Input: part model. Units: mm. Frame: model coordinates. Face numbers are marked on the shaded views. Give positions to 0.01 mm unless a question says otherwise; leave off trailing zeros. Write each loop counter-clockwise with the first axis right and the second up, starting at its lowest first coordinate (ties: lowest second). Pieces come first, ordered by that corner, then holes. Notation, with made-up numbers: (56, -8) -> (96, -8) arc R18 ccw to (96, 0) -> close; hole circle Ø8 at (-40, -22.5). An arc over 180 degrees is marked (long way). Answer as a JSON object with one key per item and string values. Group by question number.
from build123d import *

# Parameters (mm, degrees)
SKETCH1_R               = 26
SKETCH1_R_2             = 23.9
BOSS_EXTRUDE1_DEPTH     = 300
SKETCH3_R               = 2.75
CUT_EXTRUDE2_DEPTH      = 27
CIRPATTERN1_COUNT       = 3
SKETCH5_R               = 2.75
CUT_EXTRUDE3_DEPTH      = 27.0000001
CUT_EXTRUDE3_DEPTH_BACK = 27.0000001


with BuildPart() as part:
    # Sketch1 → Boss-Extrude1 (new body)
    with BuildSketch(Plane(origin=(0, 0, 0), x_dir=(1, 0, 0), z_dir=(0, 1, 0))):
        Circle(SKETCH1_R)
        Circle(SKETCH1_R_2, mode=Mode.SUBTRACT)
    extrude(amount=BOSS_EXTRUDE1_DEPTH)

    # Sketch3 → Cut-Extrude2 (cut, through all)
    with BuildSketch(Plane.XY):
        with Locations((0, 6)):
            Circle(SKETCH3_R)
        with Locations((0, 187)):
            Circle(SKETCH3_R)
    cut_extrude2 = extrude(amount=-CUT_EXTRUDE2_DEPTH, mode=Mode.SUBTRACT)

    # CirPattern1: Cut-Extrude2 ×3 about axis
    cirpattern1_axis = Axis((0, 300, 0), (0, -1, 0))
    for i in range(1, CIRPATTERN1_COUNT):
        add(cut_extrude2.rotate(cirpattern1_axis, i * 360 / CIRPATTERN1_COUNT), mode=Mode.SUBTRACT)

    # Sketch5 → Cut-Extrude3 (cut, two sides)
    with BuildSketch(Plane(origin=(0, 0, 0), x_dir=(0, 0, -1), z_dir=(1, 0, 0))) as cut_extrude3_sk:
        with Locations((0, 187)):
            Circle(SKETCH5_R)
        with Locations((0, 6)):
            Circle(SKETCH5_R)
    extrude(amount=CUT_EXTRUDE3_DEPTH, mode=Mode.SUBTRACT)
    extrude(cut_extrude3_sk.sketch, amount=-CUT_EXTRUDE3_DEPTH_BACK, mode=Mode.SUBTRACT)


solid = part.part
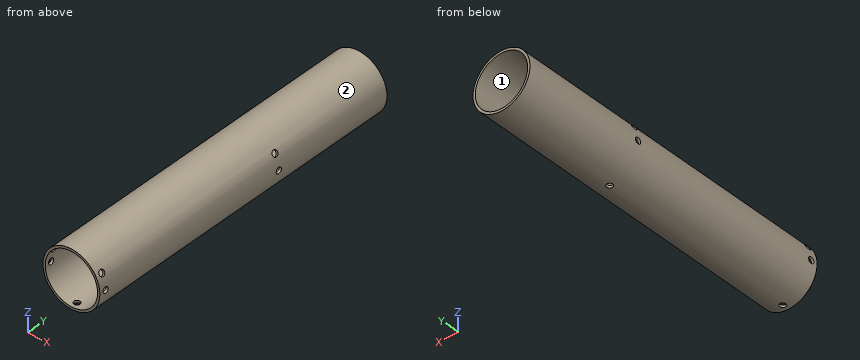
1. Line query: line 1 (Y direction, x = 0, z = -25.4); line 2 (X direction, y = 164, z = 0). Output: solid intervals per line, ascending.
2. Section D-D (z = -11). Return the cut outline in (x, y), plus the area to 3 significant figures.
3. Section C-C (y = 187). Return the cut outline in (x, z), plus the area to 3 significant figures.
4. Mould query, pull axis X, two halves, no side actions, for the marked faces 1 and 2. Classes: pulls with the +X half, pulls with the -X half, needs draft (parallel to the pull), parting line crosses it, or undercut.
5. Contact query for flat-ended pins moving along their axis: pin 1 Ø9 at (x, y) = (0, 187) entering from +Z; pin 2 Ø6.5 at (y, z) = (187, 0) entering from -X; pin 3 Ø6 at (y, z) = (127, 5) entering from +X; pin 4 Ø1 at (x, y) = (18.5, 215.5) entering from -Z. Output: stop coordinate, or through.
6. Section A-A (x = 0). Return the cut outline in (y, z).
7. Section B-B (z = 0). Return the cut outline in (x, y).
Working result:
{
 "1": {"line 1": "y = 0 to 3.25, 8.75 to 184.25, 189.75 to 300", "line 2": "x = -26 to -23.9, 23.9 to 26"},
 "2": {"outline": "(-23.56, 0) -> (-21.22, 0) -> (-21.22, 300) -> (-23.56, 300) -> close; (21.22, 0) -> (23.56, 0) -> (23.56, 300) -> (21.22, 300) -> close", "area": "1,400 mm^2"},
 "3": {"outline": "(-25.85, -2.75) arc R26 ccw to (-2.75, -25.85) -> (-2.75, -23.74) arc R23.9 cw to (-23.74, -2.75) -> close; (-25.85, 2.75) -> (-23.74, 2.75) arc R23.9 cw to (-21.94, 9.49) -> (-23.77, 10.55) arc R26 ccw to start; (-21.02, 15.31) -> (-19.19, 14.25) arc R23.9 cw to (19.19, 14.25) -> (21.02, 15.31) arc R26 ccw to start; (2.75, -25.85) arc R26 ccw to (25.85, -2.75) -> (23.74, -2.75) arc R23.9 cw to (2.75, -23.74) -> close; (21.94, 9.49) arc R23.9 cw to (23.74, 2.75) -> (25.85, 2.75) arc R26 ccw to (23.77, 10.55) -> close", "area": "271 mm^2"},
 "4": {"face 1": "undercut", "face 2": "parting line crosses it"},
 "5": {"pin 1": "stops at z = 26", "pin 2": "stops at x = -26", "pin 3": "stops at x = 25.92", "pin 4": "stops at z = -18.76"},
 "6": {"outline": "(0, -26) -> (3.25, -26) -> (3.25, -23.9) -> (0, -23.9) -> close; (0, 23.9) -> (300, 23.9) -> (300, 26) -> (0, 26) -> close; (8.75, -26) -> (184.25, -26) -> (184.25, -23.9) -> (8.75, -23.9) -> close; (189.75, -26) -> (300, -26) -> (300, -23.9) -> (189.75, -23.9) -> close"},
 "7": {"outline": "(-26, 0) -> (-23.9, 0) -> (-23.9, 3.25) -> (-26, 3.25) -> close; (-26, 8.75) -> (-23.9, 8.75) -> (-23.9, 184.25) -> (-26, 184.25) -> close; (-26, 189.75) -> (-23.9, 189.75) -> (-23.9, 300) -> (-26, 300) -> close; (23.9, 0) -> (26, 0) -> (26, 3.25) -> (23.9, 3.25) -> close; (23.9, 8.75) -> (26, 8.75) -> (26, 184.25) -> (23.9, 184.25) -> close; (23.9, 189.75) -> (26, 189.75) -> (26, 300) -> (23.9, 300) -> close"}
}
